Source: CAD feature listing. Evaluate the final solid. Frame: model axes, mm. A direction names the side the tool comes from. Coordinates: 2 decimals unless noted, no trailing zeros. Loops run counter-clockwise (first coordinate to the right, second up) from the corner with the lowest first, then second, coordinate; pieces in that order, holes last. Notation, with made-up numbers: (28.5, 12) -> (73.5, 12) arc R31 ccw to (73.5, 40) -> close; hole circle Ø3 at (31, 81.5). An arc over 180 degrees is marked (long way). Answer as CSV lines item,"result".
from build123d import *

# Parameters (mm, degrees)
F0_W     = 65
F0_H     = 50
F1_DEPTH = 2
F2_W     = 10
F2_H     = 15
F3_DEPTH = 20
F4_R     = 1
F5_DEPTH = 5
F6_R     = 1
F7_DEPTH = 25


with BuildPart() as f1:
    # F0 (on Top) → F1 (new body)
    with BuildSketch(Plane.XY):
        with Locations((32.5, 25)):
            Rectangle(F0_W, F0_H)
    extrude(amount=F1_DEPTH)

    # F2 (on face) → F3 (join)
    with BuildSketch(Plane.XY.offset(2)):
        with Locations((5, 17.5)):
            Rectangle(F2_W, F2_H)
        with Locations((60, 17.5)):
            Rectangle(F2_W, F2_H)
    extrude(amount=F3_DEPTH)

    # F4 (on face) → F5 (cut)
    with BuildSketch(Plane.XZ.offset(-10)):
        with Locations((5, 17)):
            Circle(F4_R)
        with Locations((5, 7)):
            Circle(F4_R)
        with Locations((60, 17)):
            Circle(F4_R)
        with Locations((60, 7)):
            Circle(F4_R)
    extrude(amount=-F5_DEPTH, mode=Mode.SUBTRACT)

    # F6 (on face) → F7 (cut)
    with BuildSketch(Plane.XY.offset(2)):
        with Locations((5, 45)):
            Circle(F6_R)
        with Locations((60, 45)):
            Circle(F6_R)
        with Locations((60, 5)):
            Circle(F6_R)
        with Locations((5, 5)):
            Circle(F6_R)
    extrude(amount=-F7_DEPTH, mode=Mode.SUBTRACT)


solid = f1.part
(1) Cut plane B-B (y = 5). Return the cut outline in (x, z), then the cut area to 3 significant figures.
Computed values:
outline,"(0, 0) -> (4, 0) -> (4, 2) -> (0, 2) -> close; (6, 0) -> (59, 0) -> (59, 2) -> (6, 2) -> close; (61, 0) -> (65, 0) -> (65, 2) -> (61, 2) -> close"
area,"122 mm^2"
(2) Cut plane D-D (y = 12.5). Return the cut outline in (x, z).
Computed values:
outline,"(0, 0) -> (65, 0) -> (65, 22) -> (55, 22) -> (55, 2) -> (10, 2) -> (10, 22) -> (0, 22) -> close; hole circle Ø2 at (5, 7); hole circle Ø2 at (5, 17); hole circle Ø2 at (60, 7); hole circle Ø2 at (60, 17)"
(3) Cut plane C-C (x = 60). Return the cut outline in (y, z).
Computed values:
outline,"(0, 0) -> (4, 0) -> (4, 2) -> (0, 2) -> close; (6, 0) -> (44, 0) -> (44, 2) -> (25, 2) -> (25, 22) -> (10, 22) -> (10, 18) -> (15, 18) -> (15, 16) -> (10, 16) -> (10, 8) -> (15, 8) -> (15, 6) -> (10, 6) -> (10, 2) -> (6, 2) -> close; (46, 0) -> (50, 0) -> (50, 2) -> (46, 2) -> close"
(4) Draft query along Y for faces 1 (the flat face through (60, 10, 12)), 2 (the cylindrical face through (59.263, 45.676, 1.014)), 3 (the flat face through (5, 25, 12)), 4 (the cylindrical face through (59, 5, 1)). Return one class per face: released by +Y, released by -Y, zero draft, split by the parting line, or undercut.
Computed values:
face 1,"released by -Y"
face 2,"undercut"
face 3,"released by +Y"
face 4,"undercut"
(5) Pin query (flat end, axial travel): pin 1 Ø0.6 at (x, z) = (5, 7) entering from -Y; pin 2 Ø10 at (y, z) = (16, 7) entering from -X; pin 3 Ø2.5 at (x, z) = (60, 7) entering from -Y; pin 4 Ø1.8 at (x, y) = (60, 45) entering from -Z. Return the tip coordinate at first contact, or that it passes through.
Computed values:
pin 1,"y = 15"
pin 2,"x = 0"
pin 3,"y = 10"
pin 4,"through"
(6) Cut plane A-A (z = 17). Return the cut outline in (x, y), then the cut area to 3 significant figures.
Computed values:
outline,"(0, 10) -> (4, 10) -> (4, 15) -> (6, 15) -> (6, 10) -> (10, 10) -> (10, 25) -> (0, 25) -> close; (55, 10) -> (59, 10) -> (59, 15) -> (61, 15) -> (61, 10) -> (65, 10) -> (65, 25) -> (55, 25) -> close"
area,"280 mm^2"
(7) Access query for faces 5 (the flat face through (60, 18, 22)), 6 (the flat face through (10, 17, 12)), 7 (the flat face through (5, 15, 17)). Directions: +Z, -Z, +X, -X, +Y, -Y. A direction counts if a zero-diameter tool reaches every point of the face in a straight line with its end or side. Return the directions, or none.
Computed values:
face 5,"+Z, +X, -X, +Y, -Y"
face 6,"+Z, +Y, -Y"
face 7,"-Y"
(8) Material intervals for L1, parallel to Z at x = 60, y = 11; L2, parallel to Y at x = 5, z = 0.5; L3, parallel to X at y = 20.5, z = 13.25, sorted ascending. Write a range as [from, to].
Computed values:
L1,"[0, 6], [8, 16], [18, 22]"
L2,"[0, 4], [6, 44], [46, 50]"
L3,"[0, 10], [55, 65]"
